For this review, take the finished solid that the model builds, in its own axes (mm). Give positions to 0.01 mm unless a question says otherwise; leave off trailing zeros. Loops run counter-clockwise (first coordinate to the right, second up) from the corner with the lowest first, then second, coordinate; pieces in that order, holes last. Notation, with made-up numbers: (78.25, -33) - (91.25, -33) arc R22 ccw to (91.25, -12) - close; hole circle Ø5 at (13.5, 83.5). An arc over 180 degrees is marked (long way). Use CSV: the item, a comma, the result in double quotes. Start each with the question number.
1. Take a section at D-D on x = 9. Give the boundary of the cut face in (y, z).
2. Wall thickness on line 1 (Z direction, x = 0, y = -0.2); line 2 (X direction, y = 0.2, z = -2.5); line 3 (X direction, y = -0.8, z = 11): over which ranges is each line inside the solid? List them lowest first.
3. Take a section at C-C on z = -3.75. Give the boundary of the cut face in (x, y), plus the area to 3 significant figures.
4. Take a section at A-A on y = 0.15. Give the boundary of the cut face in (x, z), plus the area to 3 significant figures.
5. For pin 1 (9 mm diameter, centred on x = 0, z = -2.5, fed in from +Y); pin 2 (1.5 mm diameter, centred on x = 1.5, z = -1.5, fed in from +Y), all flat-tipped, find the tip position at first contact; note any pin that passes through.
6. Mouldability with a two-part tool opening along Z and no side actions: class faces 1 (the flat face through (2, 0, 12.5)), 2 (the flat face through (0, 0, -12.5)), 3 (the cylindrical face through (-0.867, -0.014, 1.405)) as pulls with the +Z half, pulls with the -Z half, needs draft (parallel to the pull), parting line crosses it, or undercut.
7. Take a section at B-B on x = 0. Give the boundary of the cut face in (y, z).
```python
from build123d import *

# Parameters (mm, degrees)
SKETCH1_R           = 4
BOSS_EXTRUDE1_DEPTH = 1
CHAMFER1_SIZE       = 4


with BuildPart() as part:
    # Sketch1 → Boss-Extrude1 (new body, symmetric)
    with BuildSketch(Plane(origin=(0, 0, 0), x_dir=(1, 0, 0), z_dir=(0, 1, 0))):
        Polygon((5, 12.5), (-5, 12.5), (-15, 2.5), (-15, -12.5), (15, -12.5), (15, 2.5), align=None)
        with Locations((0, 2.5)):
            Circle(SKETCH1_R, mode=Mode.SUBTRACT)
    extrude(amount=BOSS_EXTRUDE1_DEPTH, both=True)

    # Chamfer1
    chamfer1_edges = [part.edges().sort_by_distance(p)[0] for p in [
        (-15, 0, 12.5),
    ]]
    chamfer(chamfer1_edges, length=CHAMFER1_SIZE)


solid = part.part
```
Check result:
1,outline,"(-1, -8.5) - (1, -8.5) - (1, 12.5) - (-1, 12.5) - close"
2,line 1,"z = -12.5 to -6.5, 1.5 to 12.5"
2,line 2,"x = -15 to -4, 4 to 15"
2,line 3,"x = -12.5 to 15"
3,outline,"(-13.75, -1) - (-3.8, -1) - (-3.8, 1) - (-13.75, 1) - close; (3.8, -1) - (13.75, -1) - (13.75, 1) - (3.8, 1) - close"
3,area,"39.8 mm²"
4,outline,"(-15, -2.5) - (-5, -12.5) - (5, -12.5) - (15, -2.5) - (15, 12.5) - (-11, 12.5) - (-15, 8.5) - close; hole circle Ø8 at (0, -2.5)"
4,area,"592 mm²"
5,pin 1,"stops at y = 1"
5,pin 2,"passes through"
6,face 1,"pulls with the +Z half"
6,face 2,"pulls with the -Z half"
6,face 3,"undercut"
7,outline,"(-1, -12.5) - (1, -12.5) - (1, -6.5) - (-1, -6.5) - close; (-1, 1.5) - (1, 1.5) - (1, 12.5) - (-1, 12.5) - close"
